Design review of the part built by this model. Coordinates are the model's own, in mm. A direction names the side the tool comes from. Coordinates: 2 decimals unless noted, no trailing zeros. Loops run counter-clockwise (first coordinate to the right, second up) from the corner with the lowest first, then second, coordinate; pieces in that order, holes last.
Q1. Add section A-A on x = 0. Give the boundary of the cut face in (y, z) (3 decimals).
Q2. For P1, Ø1.7, axis at x = 11, z = 45.5, coming from the +Y side; P2, Ø2.5, axis at x = 11.5, z = 41, coming from the -Y side; P3, Ø1.7, axis at x = -10.5, z = 48, coming from the -Y side, all flat-tipped, find the tip position at first contact; note any pin that passes through.
Q3. Add section B-B on y = 0. Give the boundary of the cut face in (x, z) (3 decimals).
Q4. Draft analysis for pull direction X (two halves, no side actions). For faces 1 (the face through (12.114, 3.815, 62.611)), 2 (the face through (-2.06, -9.3, 62.61)), 3 (the face through (5, 9, 0)), state which applies: released by +X, released by -X, zero draft, split by the parting line, or undercut.
Q5. Add section D-D on x = 10.75. Give the boundary of the cut face in (y, z).
Q6. Add section C-C on z = 48. Give the boundary of the cut face in (x, y) (3 decimals), and give its area (3 significant figures).
Q7. Wall thickness on probe 1 along Y at (x, z) = (0, 34) (3 decimals); probe 2 along Z at (x, y) = (10.75, 0.25): over which ranges is each line inside the solid? List them lowest first.
Q8. Machinability: for faces 4 (the face through (5, 9, 127)), 5 (the face through (10.798, -0.072, 57.327)), which of the approach directions +Z, -Z, +X, -X, +Y, -Y give a long, thin tool a straight path to every point of the face, cutting with its end or side? Answer none if there is none.
```python
from build123d import *

# Parameters (mm, degrees)
SKETCH1_R               = 12.7
SKETCH1_R_2             = 9.525
BOSS_EXTRUDE1_DEPTH     = 127
CUT_EXTRUDE1_DEPTH      = 129.263712717
CUT_EXTRUDE1_DEPTH_BACK = 129.263712717


with BuildPart() as part:
    # Sketch1 → Boss-Extrude1 (new body)
    with BuildSketch(Plane.XY):
        Circle(SKETCH1_R)
        Circle(SKETCH1_R_2, mode=Mode.SUBTRACT)
    extrude(amount=BOSS_EXTRUDE1_DEPTH)

    # Sketch2 → Cut-Extrude1 (cut, two sides: drawn at the far end of the back side and taken through both)
    with BuildSketch(Plane(origin=(0, 0, 0), x_dir=(0, 0, -1), z_dir=(1, 0, 0)).offset(-CUT_EXTRUDE1_DEPTH_BACK)):
        with BuildLine():
            Line((-35.0139, -3.2639), (-54.0639, -3.2639))
            ThreePointArc((-54.0639, -3.2639), (-57.3278, 0), (-54.0639, 3.2639))
            Line((-54.0639, 3.2639), (-35.0139, 3.2639))
            ThreePointArc((-35.0139, 3.2639), (-31.75, 0), (-35.0139, -3.2639))
        make_face()
    extrude(amount=CUT_EXTRUDE1_DEPTH + CUT_EXTRUDE1_DEPTH_BACK, mode=Mode.SUBTRACT)


solid = part.part
```
Entries:
1. outline: (-12.7, 0) - (-9.525, 0) - (-9.525, 127) - (-12.7, 127) - close; (9.525, 0) - (12.7, 0) - (12.7, 127) - (9.525, 127) - close
2. P1: stops at y = 7.63
2. P2: stops at y = -7.5
2. P3: stops at y = -8.26
3. outline: (-12.7, 0) - (-9.525, 0) - (-9.525, 31.75) - (-12.7, 31.75) - close; (-12.7, 57.328) - (-9.525, 57.328) - (-9.525, 127) - (-12.7, 127) - close; (9.525, 0) - (12.7, 0) - (12.7, 31.75) - (9.525, 31.75) - close; (9.525, 57.328) - (12.7, 57.328) - (12.7, 127) - (9.525, 127) - close
4. face 1: split by the parting line
4. face 2: undercut
4. face 3: zero draft
5. outline: (-6.76, 0) - (6.76, 0) - (6.76, 127) - (-6.76, 127) - close; hole (-3.26, 35.01) arc R3.26 ccw to (3.26, 35.01) - (3.26, 54.06) arc R3.26 ccw to (-3.26, 54.06) - close
6. outline: (-12.273, -3.264) arc R12.7 ccw to (12.273, -3.264) - (8.948, -3.264) arc R9.525 cw to (-8.948, -3.264) - close; (-12.273, 3.264) - (-8.948, 3.264) arc R9.525 cw to (8.948, 3.264) - (12.273, 3.264) arc R12.7 ccw to start
6. area: 180 mm2
7. probe 1: y = -12.7 to -9.525, 9.525 to 12.7
7. probe 2: z = 0 to 31.76, 57.32 to 127
8. face 4: +Z, +X, -X, +Y, -Y
8. face 5: +X, -X
